```python
from build123d import *

# Parameters (mm, degrees)
SKETCH_W     = 40
SKETCH_H     = 25
PAD_DEPTH    = 6
POCKET_DEPTH = 4
FILLET_R     = 1
FILLET001_R  = 1


with BuildPart() as part:
    # Sketch → Pad (new body)
    with BuildSketch(Plane.XY):
        Rectangle(SKETCH_W, SKETCH_H)
    extrude(amount=PAD_DEPTH)

    # Sketch001 → Pocket (cut)
    with BuildSketch(Plane.XY.offset(6)):
        with BuildLine():
            ThreePointArc((-11.3, 2.8), (-14.1, 0), (-11.3, -2.8))
            Line((-11.3, -2.8), (-8.5, -2.8))
            ThreePointArc((-8.5, -2.8), (-5.7, 0), (-8.5, 2.8))
            Line((-11.3, 2.8), (-8.5, 2.8))
        make_face()
    extrude(amount=-POCKET_DEPTH, mode=Mode.SUBTRACT)

    # Fillet
    fillet_edges = [part.edges().sort_by_distance(p)[0] for p in [
        (-20, 0, 0),
        (0, 12.5, 0),
        (0, -12.5, 0),
        (20, 0, 0),
    ]]
    fillet(fillet_edges, radius=FILLET_R)

    # Fillet001
    fillet001_edges = [part.edges().sort_by_distance(p)[0] for p in [
        (0, -12.5, 6),
        (-20, 0, 6),
        (0, 12.5, 6),
        (20, 0, 6),
    ]]
    fillet(fillet001_edges, radius=FILLET001_R)


solid = part.part
```
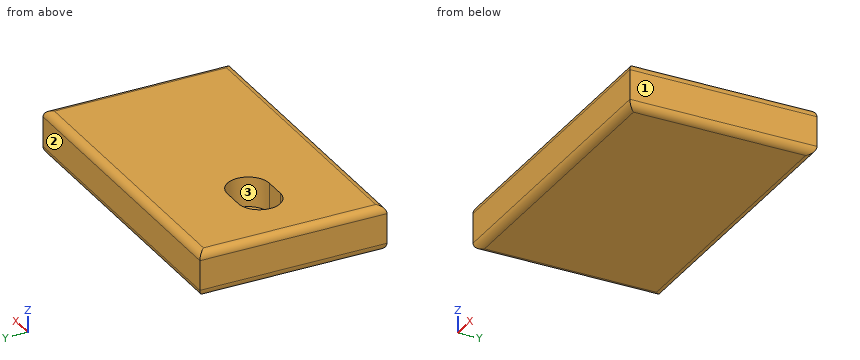
Input: part model. Units: mm. Frame: model coordinates. Face numbers are marked on the shaded views. Coordinates: 2 decimals unless noted, no trailing zeros. Order: outer loops, then holes, each group sorted by start corner. A loop starts at its lowest first (then second) coordinate and runs counter-clockwise, first axis right, second up. Notation, with made-up numbers: (51, -34.75) - (59, -34.75) arc R38 ccw to (59, 3.25) - close; hole circle Ø3 at (3, -39). An arc over 180 degrees is marked (long way). Put each result on its own line as item: value.
1. Cut plane C-C on x = -13.5. Return the cut outline in (y, z).
Report:
outline: (-12.5, 1) arc R1 ccw to (-11.5, 0) - (11.5, 0) arc R1 ccw to (12.5, 1) - (12.5, 5) arc R1 ccw to (11.5, 6) - (1.73, 6) - (1.73, 2) - (-1.73, 2) - (-1.73, 6) - (-11.5, 6) arc R1 ccw to (-12.5, 5) - close
2. Draft query along Y for the marked faces 1, 2 and 3. Return one class per face: pulls with the +Y half, pulls with the -Y half, needs draft (parallel to the pull), parting line crosses it, or undercut.
Report:
face 1: needs draft
face 2: pulls with the +Y half
face 3: undercut
3. Line query: line 1 along Y through (x, z) = (-9, 3.55); line 2 along Y through (x, z) = (-13, 3.5); line 3 along Y through (x, z) = (-0.5, 5.1). Output: solid intervals per line, ascending.
Report:
line 1: y = -12.5 to -2.8, 2.8 to 12.5
line 2: y = -12.5 to -2.22, 2.22 to 12.5
line 3: y = -12.49 to 12.49
4. Cut plane B-B on y = 0. Return the cut outline in (x, z).
Report:
outline: (-20, 1) arc R1 ccw to (-19, 0) - (19, 0) arc R1 ccw to (20, 1) - (20, 5) arc R1 ccw to (19, 6) - (-5.7, 6) - (-5.7, 2) - (-14.1, 2) - (-14.1, 6) - (-19, 6) arc R1 ccw to (-20, 5) - close
5. Cut plane A-A on z = 4.4. Return the cut outline in (x, y), then the cut area to 3 significant figures.
Report:
outline: (-20, -12.5) - (20, -12.5) - (20, 12.5) - (-20, 12.5) - close; hole (-11.3, -2.8) - (-8.5, -2.8) arc R2.8 ccw to (-8.5, 2.8) - (-11.3, 2.8) arc R2.8 ccw to start
area: 960 mm2
